Source: three-view drawing plus pictorial views. Frame: mm from the lowest corner of the part. A direction names the side the tool comes from. Coordinates: 2 decimals unless noted, no trailing zeros. Order: outer loops, then holes, each group sorted by start corner. A loop starts at its lowest first (then second) coordinate and runs counter-clockwise, first axis right, second up. Notation, with made-up numbers: (-12.75, 64.5) - (34.25, 64.5) arc R28 cw to (34.25, 92.5) - close; hole circle Ø7 at (65.25, 83). An arc over 180 degrees is marked (long way). Use a Markdown table: item, result. Add a question column.
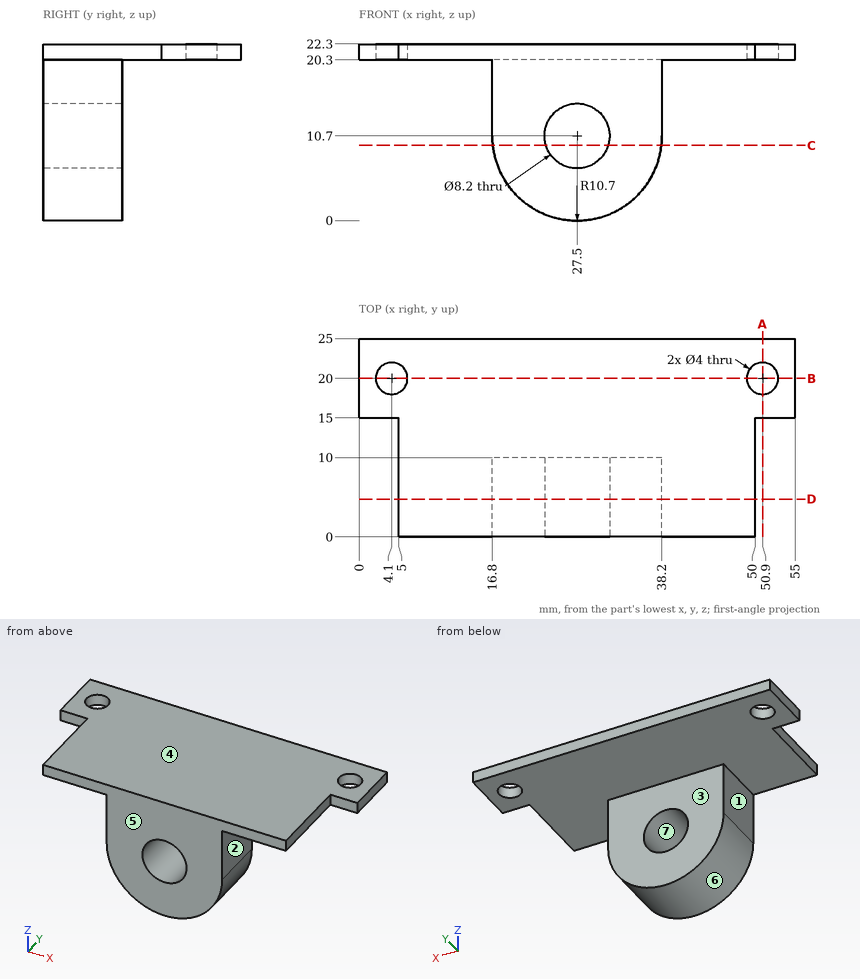
1) Draft query along Z for the marked faces 5, 6 and 7. Return one class per face: pulls with the +Z half, pulls with the -Z half, needs draft (parallel to the pull), parting line crosses it, or undercut.
2) Section C-C (z = 9.5). Return loops of the section in (x, y), then the cut area to 3 significant figures.
3) Pin query (flat end, axial travel): pin 1 (10.5 mm diameter, centred on y = 3.5, z = 17, fed in from +X); pin 2 (8 mm diameter, centred on x = 44.5, y = 15, fed in from -Z); pin 3 (1 mm diameter, centred on y = 6.5, z = 21, fed in from -X). Return the tip coordinate at first contact, or that it passes through.
4) Section D-D (y = 4.75). Return loops of the section in (x, z), then the cut area to 3 significant figures.
5) Set-up query: the marked faces 1, 2, 3 and 4. Return all of +Z, -Z, +X, -X, +Y, -Y with unobstructed straight access to the full face (end or side cutting, diameter ignored); none if empty.
6) Section A-A (x = 50.9). Return loops of the section in (y, z), then the cut area to 3 significant figures.
7) Ray query, line 1 along X through (y, z) = (20, 21.5); line 2 along X through (y, z) = (3.75, 10.7); line 3 along Z through (x, y) = (34.5, 14.5). Return the intervals inside material, ascending.
8) Section B-B (y = 20). Return loops of the section in (x, z), then the cut area to 3 significant figures.
Values follow:
| question | item | result |
|---|---|---|
| 1 | face 5 | needs draft |
| 1 | face 6 | pulls with the -Z half |
| 1 | face 7 | undercut |
| 2 | outline | (16.87, 0) - (23.58, 0) - (23.58, 10) - (16.87, 10) - close; (31.42, 0) - (38.13, 0) - (38.13, 10) - (31.42, 10) - close |
| 2 | area | 134 mm² |
| 3 | pin 1 | stops at x = 50 |
| 3 | pin 2 | stops at z = 20.3 |
| 3 | pin 3 | stops at x = 5 |
| 4 | outline | (5, 20.3) - (16.8, 20.3) - (16.8, 10.7) arc R10.7 ccw to (38.2, 10.7) - (38.2, 20.3) - (50, 20.3) - (50, 22.3) - (5, 22.3) - close; hole circle Ø8.2 at (27.5, 10.7) |
| 4 | area | 422 mm² |
| 5 | face 1 | -Z, -X, +Y, -Y |
| 5 | face 2 | -Z, +X, +Y, -Y |
| 5 | face 3 | -Z, +X, -X, +Y |
| 5 | face 4 | +Z, +X, -X, +Y, -Y |
| 6 | outline | (15, 20.3) - (18, 20.3) - (18, 22.3) - (15, 22.3) - close; (22, 20.3) - (25, 20.3) - (25, 22.3) - (22, 22.3) - close |
| 6 | area | 12.0 mm² |
| 7 | line 1 | x = 0 to 2.1, 6.1 to 48.9, 52.9 to 55 |
| 7 | line 2 | x = 16.8 to 23.4, 31.6 to 38.2 |
| 7 | line 3 | z = 20.3 to 22.3 |
| 8 | outline | (0, 20.3) - (2.1, 20.3) - (2.1, 22.3) - (0, 22.3) - close; (6.1, 20.3) - (48.9, 20.3) - (48.9, 22.3) - (6.1, 22.3) - close; (52.9, 20.3) - (55, 20.3) - (55, 22.3) - (52.9, 22.3) - close |
| 8 | area | 94.0 mm² |
